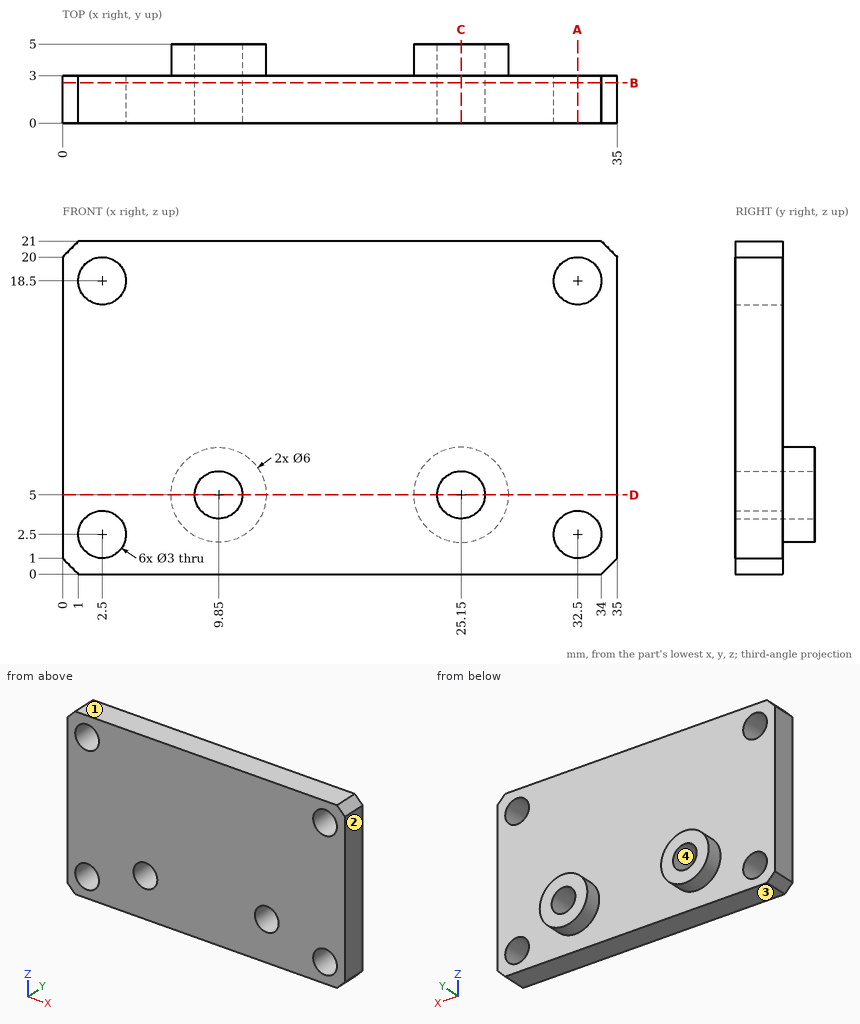
Geometry check sheet. Reference: drawing and pictorial views, mm from the part's lowest x, y, z. Give positions to 0.01 mm unless a question says otherwise; leave off trailing zeros. Loops run counter-clockwise (first coordinate to the right, second up) from the corner with the lowest first, then second, coordinate; pieces in that order, holes last. Notation, with made-up numbers: (-35, 45.5) - (2, 45.5) arc R27 ccw to (2, 61.5) - close; hole circle Ø8 at (48, 7). An arc over 180 degrees is marked (long way). Use CSV: the item, a comma, the result in double quotes. Start each with the question number.
Q1. Go/stop test with flat-tipped pins: pin 1 Ø12 at (x, z) = (15, 15.5) entering from +Y; pin 2 Ø10 at (x, z) = (30.5, 7) entering from +Y. Record where each tip stops, or that it passes through.
Q2. Section check C-C, the plane x = 25.15. Record the cut outline in (y, z), and give its area (3 significant figures).
Q3. Release check for a two-part mould opening along Z. For the marked faces 1, 2, 3 and 4 record: +Z half, -Z half, draft (parallel to the pull), parting line (faces both ways), or undercut.
Q4. Section check D-D, the plane z = 5. Record the cut outline in (x, y), and give its area (3 significant figures).
Q5. Section check B-B, the plane y = 2.55. Record the cut outline in (x, z).
Q6. Section check A-A, the plane x = 32.5. Record the cut outline in (y, z).
Q7. Scan lines: probe 1 along Z at (x, y) = (32.5, 1.4); probe 2 along X at (y, z) = (1.3, 18.5); probe 3 along X at (y, z) = (1.1, 5). Record each from-to range of solid material in increasing order. Write a range as from..to.
Findings below:
1,pin 1,"stops at y = 3"
1,pin 2,"stops at y = 5"
2,outline,"(0, 0) - (3, 0) - (3, 2) - (5, 2) - (5, 3.5) - (0, 3.5) - close; (0, 6.5) - (5, 6.5) - (5, 8) - (3, 8) - (3, 21) - (0, 21) - close"
2,area,"60.0 mm^2"
3,face 1,"+Z half"
3,face 2,"draft"
3,face 3,"-Z half"
3,face 4,"undercut"
4,outline,"(0, 0) - (8.35, 0) - (8.35, 5) - (6.85, 5) - (6.85, 3) - (0, 3) - close; (11.35, 0) - (23.65, 0) - (23.65, 5) - (22.15, 5) - (22.15, 3) - (12.85, 3) - (12.85, 5) - (11.35, 5) - close; (26.65, 0) - (35, 0) - (35, 3) - (28.15, 3) - (28.15, 5) - (26.65, 5) - close"
4,area,"99.0 mm^2"
5,outline,"(0, 1) - (1, 0) - (34, 0) - (35, 1) - (35, 20) - (34, 21) - (1, 21) - (0, 20) - close; hole circle Ø3 at (2.5, 2.5); hole circle Ø3 at (2.5, 18.5); hole circle Ø3 at (9.85, 5); hole circle Ø3 at (25.15, 5); hole circle Ø3 at (32.5, 2.5); hole circle Ø3 at (32.5, 18.5)"
6,outline,"(0, 0) - (3, 0) - (3, 1) - (0, 1) - close; (0, 4) - (3, 4) - (3, 17) - (0, 17) - close; (0, 20) - (3, 20) - (3, 21) - (0, 21) - close"
7,probe 1,"z = 0..1, 4..17, 20..21"
7,probe 2,"x = 0..1, 4..31, 34..35"
7,probe 3,"x = 0..8.35, 11.35..23.65, 26.65..35"
